The figure shows three views and two pictorial views of one solid part (mm, origin at its lowest corner). Answer the questions. Round coordinates to 2 decimals unless told otherwise and drop trailing zeros. Write each loop counter-clockwise with the first axis right and the second up, starting at its lowest first coordinate (ties: lowest second). Pieces come first, ordered by that corner, then holes. Notation, with made-up numbers: (89, 3) - (135, 3) arc R19 ccw to (135, 17) - close; hole circle Ø1 at (-12, 59.25). An arc over 180 degrees is marked (long way). Answer as CSV lines item,"result". Start each with the question number.
Item 1: A cutting plane is placed at B-B on y = 1.5. Determine the outline of the cut face in (x, z) (1 decimal).
Item 2: Straight lines are drawn through the part: line 1 along X through (y, z) = (4.5, 155); line 2 along Z through (x, y) = (279, 2.25) (1 decimal). For each, find the intervals that lie inside material, in ascending order. Write a range as [from, to].
Item 3: A cutting plane is placed at A-A on z = 171. Determine the outline of the cut face in (x, y), and give its area (3 significant figures).
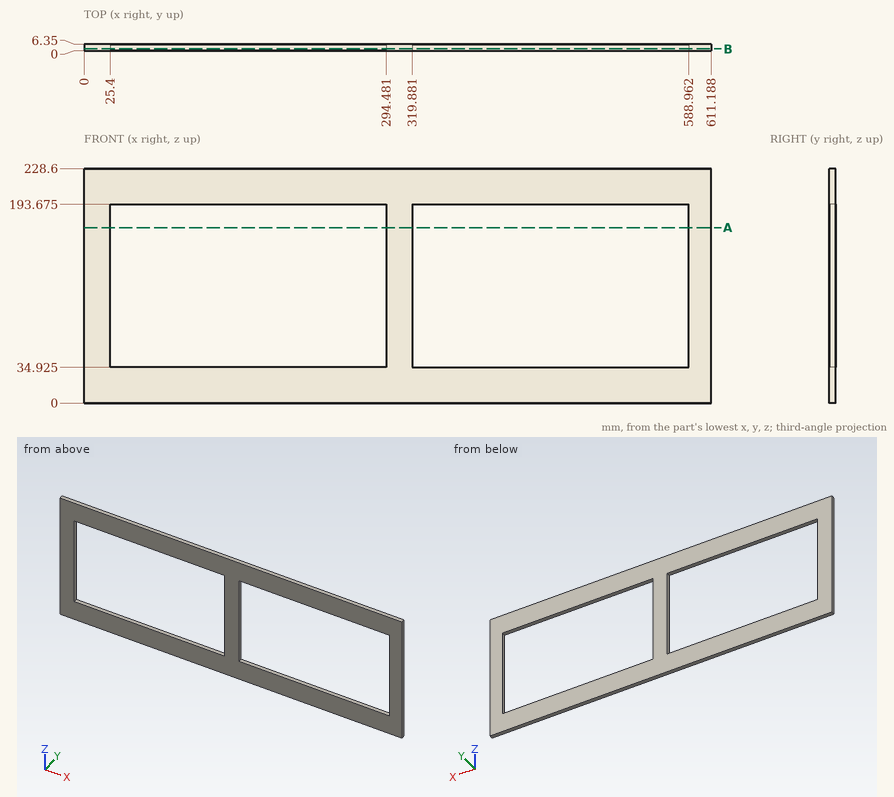
Geometry says:
1,outline,"(0, 0) - (611.2, 0) - (611.2, 228.6) - (0, 228.6) - close; hole (25.4, 34.9) - (294.5, 34.9) - (294.5, 193.7) - (25.4, 193.7) - close; hole (319.9, 34.9) - (589, 34.9) - (589, 193.7) - (319.9, 193.7) - close"
2,line 1,"x = [0, 25.4], [294.48, 319.88], [588.96, 611.19]"
2,line 2,"z = [0, 34.9], [193.7, 228.6]"
3,outline,"(0, 0) - (25.4, 0) - (25.4, 6.35) - (0, 6.35) - close; (294.48, 0) - (319.88, 0) - (319.88, 6.35) - (294.48, 6.35) - close; (588.96, 0) - (611.19, 0) - (611.19, 6.35) - (588.96, 6.35) - close"
3,area,"464 mm^2"
